Autodesk Inventor part; units mm, degrees
ref_plane "YZ Plane" through (0, 0, 0) normal (1, 0, 0) x (0, 1, 0)
ref_plane "XZ Plane" through (0, 0, 0) normal (0, 1, 0) x (-1, 0, 0)
ref_plane "XY Plane" through (0, 0, 0) normal (0, 0, 1) x (1, 0, 0)
sketch "Sketch1" plane through (0, 0, 0) normal (0, 1, 0) x (-1, 0, 0)
  line L0 (0, 0) -> (-111.76, 0)
  line L1 (-111.76, 0) -> (-111.76, 215.9)
  line L2 (-111.76, 215.9) -> (0, 215.9)
  line L3 (0, 215.9) -> (0, 0)
  dimension "d0" = 111.76
  dimension "d1" = 215.9
extrude "Extrusion1" add sketch "Sketch1" along normal blind 91.44
shell "Shell1" thickness 3.81 removed faces 1 at (37.2533, 91.44, 71.9667)
sketch "Sketch2" plane through (0, 0, 215.9) normal (0, 0, 1) x (1, 0, 0)
  line L0 (0, 0) -> (111.76, 0)
  line L1 (111.76, 0) -> (111.76, 91.44)
  line L2 (0, 91.44) -> (111.76, 91.44)
  line L3 (0, 0) -> (0, 91.44)
  point P0 (0, 0)
extrude "Extrusion2" cut sketch "Sketch2" against normal up to surface (3.81 mm away)
sketch "Sketch3" plane through (0, 0, 0) normal (0, -1, 0) x (1, 0, 0)
  line L0 (111.76, 212.09) -> (0, 212.09)
  line L1 (0, 0) -> (0, 212.09)
  line L2 (111.76, 212.09) -> (111.76, 0)
  line L3 (111.76, 212.09) -> (0, 212.09)
  line L4 (0, 0) -> (0, 212.09)
  line L5 (111.76, 0) -> (0, 0)
  line L6 (111.76, 212.09) -> (111.76, 0)
  line L7 (111.76, 212.09) -> (111.76, 0)
  line L8 (0, 0) -> (0, 212.09)
  spline S0 degree 4 poles (111.76, 85.3366) (95.0927, 139.8259) (66.5153, -13.509) (18.6749, 203.0999) (15.6726, 63.615) (0, 106.045) knots 0 0 0 0 0 0.532853 1 1 1 1 1
  point P0 (85.9461, 95.2827)
  point P1 (57.1117, 86.6573)
  point P2 (28.3059, 111.5489)
  point P3 (15.0905, 97.7863)
  point P4 (0, 106.045)
  point P5 (111.76, 85.3366)
sketch "Sketch4" plane through (0, 91.44, 0) normal (0, 1, 0) x (1, 0, 0)
  line L0 (3.81, -212.09) -> (3.81, -3.81)
  line L1 (3.81, -3.81) -> (107.95, -3.81)
  line L2 (107.95, -3.81) -> (107.95, -212.09)
  line L3 (107.95, -3.81) -> (3.81, -3.81)
  line L4 (3.81, -3.81) -> (13.81, -3.81)
  line L5 (13.81, -3.81) -> (13.81, -13.81)
  line L6 (13.81, -13.81) -> (3.81, -13.81)
  line L7 (3.81, -13.81) -> (3.81, -3.81)
  line L8 (107.95, -3.81) -> (97.95, -3.81)
  line L9 (97.95, -3.81) -> (97.95, -13.81)
  line L10 (97.95, -13.81) -> (107.95, -13.81)
  line L11 (107.95, -13.81) -> (107.95, -3.81)
  line L12 (107.95, -212.09) -> (107.95, -3.81)
  line L13 (107.95, -212.09) -> (97.95, -212.09)
  line L14 (97.95, -212.09) -> (97.95, -202.09)
  line L15 (97.95, -202.09) -> (107.95, -202.09)
  line L16 (107.95, -202.09) -> (107.95, -212.09)
  line L17 (3.81, -212.09) -> (13.81, -212.09)
  line L18 (13.81, -212.09) -> (13.81, -202.09)
  line L19 (13.81, -202.09) -> (3.81, -202.09)
  line L20 (3.81, -202.09) -> (3.81, -212.09)
  point P0 (3.81, -202.09)
  point P1 (97.95, -3.81)
  dimension "d9" = 10
  dimension "d10" = 10
  dimension "d11" = 10
  dimension "d12" = 10
  dimension "d13" = 10
  dimension "d14" = 10
  dimension "d15" = 10
  dimension "d16" = 10
extrude "Extrusion4" add sketch "Sketch4" against normal blind 30
sketch "Sketch5" plane through (0, 91.44, 0) normal (0, 1, 0) x (1, 0, 0)
  circle A0 centre (8.81, -8.81) radius 2
  circle A1 centre (105.49, -8.81) radius 2
  circle A2 centre (105.49, -207.09) radius 2
  circle A3 centre (8.81, -207.09) radius 2
  dimension "d19" = 4
  dimension "d20" = 4
  dimension "d21" = 4
  dimension "d22" = 4
extrude "Extrusion5" cut sketch "Sketch5" against normal blind 15
The listing builds one solid part. Answer for the finished solid, in the listing's coordinates (mm). A direction names the side the tool comes from. Coordinates: 2 decimals unless noted, no trailing zeros. Write each loop counter-clockwise with the first axis right and the second up, starting at its lowest first coordinate (ties: lowest second). Pieces come first, ordered by that corner, then holes. Notation, with made-up numbers: M 56.5,13.5 L 63.5,13.5 A18 cw 63.5,21.5 Z; hole C 17,29.25 d6. An arc over 180 degrees is marked long. Use a Markdown table: item, result. Add a question column.
1. Section A-A (z = 32.5) is taken. Give the vertices of the cut face in (x, y).
2. For a pull along Z with two mould halves and no side action, classify faces 1 (the flat face through (57, 3.81, 109)), 2 (the flat face through (56, 2, 212.09)), 3 (the flat face through (9, 76.44, 207)) as +Z half, -Z half, draft (parallel to the pull), parting line (faces both ways), or undercut.
3. Section C-C (x = 45) is taken. Give the vertices of the cut face in (y, z).
4. Given P1, Ø5, axis at x = 80, z = 42, coming from the +Y side, flat-ended and moving along its own axis, determine where the tip first touches the part or whether it passes through.
5. Which of the six approach directions +Z, -Z, +X, -X, +Y, -Y give full straight-line access (tool end or side, diameter ignored) to faces 4 (the flat face through (0, 45, 108)), 5 (the flat face through (103, 77, 202.09)), 6 (the flat face through (103, 61.44, 9)), 7 (the flat face through (13.81, 77, 207))?
6. Straight lines are drawn through the part: line 1 along X through (y, z) = (86.75, 8.81); line 2 along Z through (x, y) = (8.81, 80.5); line 3 along X through (y, z) = (15, 145). For each, find the intervals that lie inside material, in ascending order. Write a range as [from, to].
7. Section B-B (y = 42.5) is taken. Give the vertices of the cut face in (x, z).
Data:
| question | item | result |
|---|---|---|
| 1 | outline | M 0,0 L 111.76,0 L 111.76,91.44 L 107.95,91.44 L 107.95,3.81 L 3.81,3.81 L 3.81,91.44 L 0,91.44 Z |
| 2 | face 1 | draft |
| 2 | face 2 | +Z half |
| 2 | face 3 | undercut |
| 3 | outline | M 0,0 L 91.44,0 L 91.44,3.81 L 3.81,3.81 L 3.81,212.09 L 0,212.09 Z |
| 4 | P1 | stops at y = 3.81 |
| 5 | face 4 | +Z, -Z, -X, +Y, -Y |
| 5 | face 5 | +Y |
| 5 | face 6 | +Z |
| 5 | face 7 | +Z, +Y |
| 6 | line 1 | x = [0, 6.81], [10.81, 13.81], [97.95, 103.49], [107.49, 111.76] |
| 6 | line 2 | z = [0, 6.81], [10.81, 13.81], [202.09, 205.09], [209.09, 212.09] |
| 6 | line 3 | x = [0, 3.81], [107.95, 111.76] |
| 7 | outline | M 0,0 L 111.76,0 L 111.76,212.09 L 107.95,212.09 L 107.95,3.81 L 3.81,3.81 L 3.81,212.09 L 0,212.09 Z |
